Here's how the part is built. I have some questions about the finished solid (model axes, mm). A direction names the side the tool comes from. Coordinates: 2 decimals unless noted, no trailing zeros. Write each loop counter-clockwise with the first axis right and the second up, starting at its lowest first coordinate (ties: lowest second). Pieces come first, ordered by that corner, then holes.
Item 1: For faces 5 (the face through (3.417, -0.393, 0.759)), 6 (the face through (7.81, -1.18, 1.73)), which set-ups out of +Z, -Z, +X, -X, +Y, -Y let a thin tool reach every point of the face, with its end or its side?
Item 2: Please list where these lines run through material, in increasing order: line 1 (X direction, y = 1.5, z = 0); line 2 (X direction, y = 0.15, z = 0); line 3 (Y direction, x = 2, z = -2) (3 decimals).
Item 3: If we mould it in two halves opening along Z, with no side actions, what happens to faces 1 (the face through (1.7, -1.625, -3.4)), 2 (the face through (2, 0.875, -2)), 3 (the face through (-2.44, 1.24, -0.54)), 4 (the face through (7.81, 1.19, 1.73))? For each: pulls with the +Z half, pulls with the -Z half, needs draft (parallel to the pull), parting line crosses it, or undercut.
Item 4: I want a section at A-A (z = 0). Please give me the cut outline in (x, y) (3 decimals), and give its area (3 significant figures).
Item 5: I'm going to push flat-ended pins straight in: P1, Ø5.5, axis at x = 0, z = -0.5, coming from the -Y side (3 decimals); P2, Ø1, axis at y = 0.5, z = -3.5, coming from the +X side. Where does each tip first touch, or does it pass through?
Item 6: I want a section at B-B (x = 0). Please give me the cut outline in (y, z) (3 decimals).
from build123d import *

# Parameters (mm, degrees)
SKETCH1_R           = 8
SKETCH1_R_2         = 3.5
BOSS_EXTRUDE1_DEPTH = 1.625
BOSS_EXTRUDE2_START = -0.75
SKETCH3_R           = 3.5
SKETCH3_R_2         = 2.5
BOSS_EXTRUDE2_DEPTH = 0.75


with BuildPart() as part:
    # Sketch1 → Boss-Extrude1 (new, symmetric)
    with BuildSketch(Plane(origin=(0, 0, 0), x_dir=(1, 0, 0), z_dir=(0, 1, 0))):
        with Locations(Location((0, 0, 0), (0, 0, 90))):
            Circle(SKETCH1_R)
        with Locations(Location((0, 0, 0), (0, 0, 90))):
            Circle(SKETCH1_R_2, mode=Mode.SUBTRACT)
    extrude(amount=BOSS_EXTRUDE1_DEPTH, both=True)

    # Sketch2 → Cut-Revolve1 (revolve, cut)
    with BuildSketch(Plane(origin=(0, 0, 0), x_dir=(0, 0, -1), z_dir=(1, 0, 0)), mode=Mode.PRIVATE) as cut_revolve1_sk:
        with BuildLine():
            Line((-8, 0.75), (-8, -0.75))
            ThreePointArc((-8, -0.75), (-7.25, 0), (-8, 0.75))
        make_face()
    revolve(cut_revolve1_sk.sketch.rotate(Axis((0, 1.625, 0), (0, -1, 0)), 180), axis=Axis((0, 1.625, 0), (0, -1, 0)), mode=Mode.SUBTRACT)

    # Sketch3 → Boss-Extrude2 (add)
    with BuildSketch(Plane(origin=(0, 1.625, 0), x_dir=(1, 0, 0), z_dir=(0, 1, 0)).offset(BOSS_EXTRUDE2_START)):
        with Locations(Location((0, 0, 0), (0, 0, 90))):
            Circle(SKETCH3_R)
        with Locations(Location((0, 0, 0), (0, 0, 270))):
            Circle(SKETCH3_R_2, mode=Mode.SUBTRACT)
    extrude(amount=BOSS_EXTRUDE2_DEPTH)


solid = part.part
Answer:
1. face 5: -Y
1. face 6: +Y, -Y
2. line 1: x = -8 to -2.5, 2.5 to 8
2. line 2: x = -7.27 to -3.5, 3.5 to 7.27
2. line 3: y = 0.875 to 1.625
3. face 1: needs draft
3. face 2: undercut
3. face 3: undercut
3. face 4: parting line crosses it
4. outline: (-8, -1.625) - (-3.5, -1.625) - (-3.5, 0.875) - (-2.5, 0.875) - (-2.5, 1.625) - (-8, 1.625) - (-8, 0.75) arc R0.75 cw to (-8, -0.75) - close; (2.5, 0.875) - (3.5, 0.875) - (3.5, -1.625) - (8, -1.625) - (8, -0.75) arc R0.75 cw to (8, 0.75) - (8, 1.625) - (2.5, 1.625) - close
4. area: 29.0 mm2
5. P1: stops at y = 0.875
5. P2: stops at x = 7.39
6. outline: (-1.625, -8) - (-0.75, -8) arc R0.75 cw to (0.75, -8) - (1.625, -8) - (1.625, -2.5) - (0.875, -2.5) - (0.875, -3.5) - (-1.625, -3.5) - close; (-1.625, 3.5) - (0.875, 3.5) - (0.875, 2.5) - (1.625, 2.5) - (1.625, 8) - (0.75, 8) arc R0.75 cw to (-0.75, 8) - (-1.625, 8) - close
